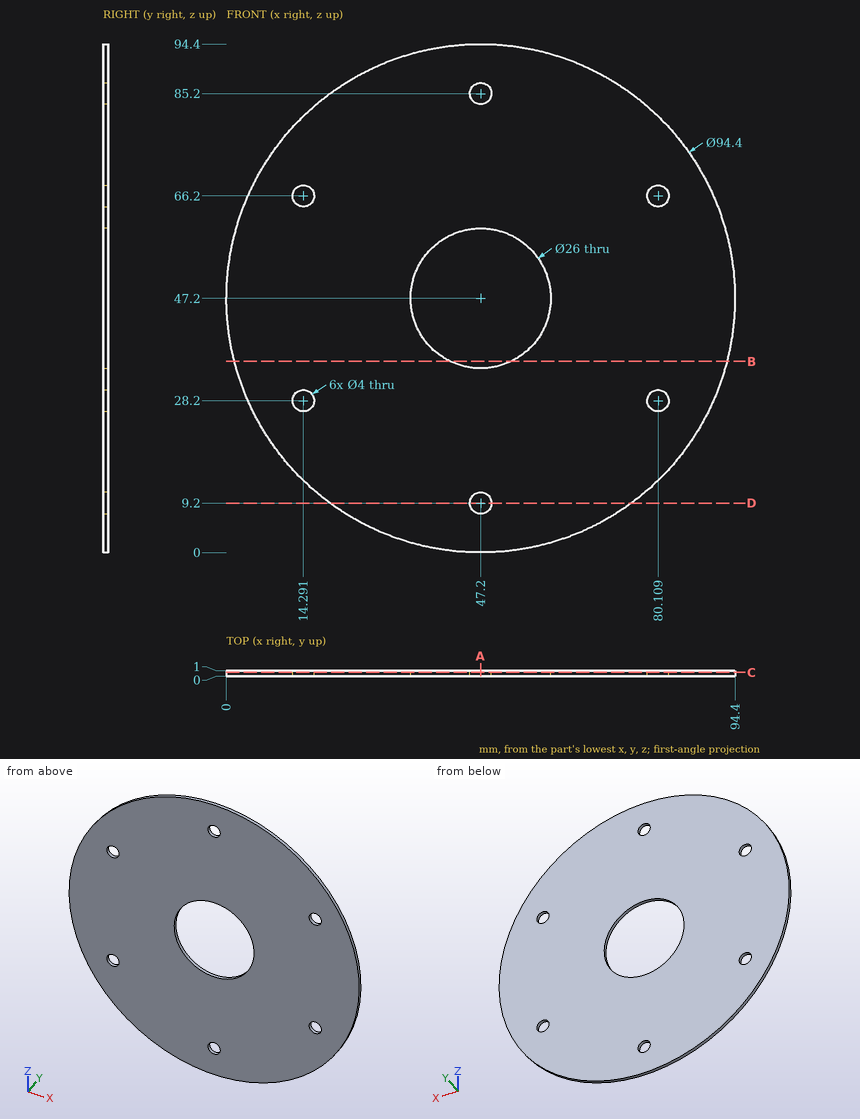
For this review, use the dimensioned drawing (mm, ordinates from the lowest corner) and the shaded views. Coordinates: 2 decimals unless noted, no trailing zeros. Loops run counter-clockwise (first coordinate to the right, second up) from the corner with the lowest first, then second, coordinate; pieces in that order, holes last. Notation, with made-up numbers: (60, 77.5) -> (88, 77.5) arc R22 cw to (88, 105.5) -> close; hole circle Ø3 at (81, 78.5). An arc over 180 degrees is marked (long way). Return JSON: item names as keys, results as strings. Group by question number.
(1) Consider section D-D, the plane z = 9.2. Give the boundary of the cut face in (x, y).
(2) Consider section A-A, the plane x = 47.2. Give the boundary of the cut face in (y, z).
(3) Consider section B-B, the plane z = 35.5. Give the boundary of the cut face in (x, y).
(4) Consider section C-C, the plane y = 0.65. Give the boundary of the cut face in (x, z).
(5) To check wall thickness, follow L1, parallel to X at y = 0.45, z = 28.2; L2, parallel to Z at x = 46.5, y = 0.6; L3, parallel to Z at x = 58, y = 0.25. State the ranges of each line that lie inside material, in increasing order.
Results below:
{
 "1": {"outline": "(19.2, 0) -> (45.2, 0) -> (45.2, 1) -> (19.2, 1) -> close; (49.2, 0) -> (75.2, 0) -> (75.2, 1) -> (49.2, 1) -> close"},
 "2": {"outline": "(0, 0) -> (1, 0) -> (1, 7.2) -> (0, 7.2) -> close; (0, 11.2) -> (1, 11.2) -> (1, 34.2) -> (0, 34.2) -> close; (0, 60.2) -> (1, 60.2) -> (1, 83.2) -> (0, 83.2) -> close; (0, 87.2) -> (1, 87.2) -> (1, 94.4) -> (0, 94.4) -> close"},
 "3": {"outline": "(1.47, 0) -> (41.53, 0) -> (41.53, 1) -> (1.47, 1) -> close; (52.87, 0) -> (92.93, 0) -> (92.93, 1) -> (52.87, 1) -> close"},
 "4": {"outline": "circle Ø94.4 at (47.2, 47.2); hole circle Ø4 at (14.29, 28.2); hole circle Ø4 at (14.29, 66.2); hole circle Ø26 at (47.2, 47.2); hole circle Ø4 at (47.2, 9.2); hole circle Ø4 at (47.2, 85.2); hole circle Ø4 at (80.11, 28.2); hole circle Ø4 at (80.11, 66.2)"},
 "5": {"L1": "x = 3.99 to 12.29, 16.29 to 78.11, 82.11 to 90.41", "L2": "z = 0.01 to 7.33, 11.07 to 34.22, 60.18 to 83.33, 87.07 to 94.39", "L3": "z = 1.25 to 39.96, 54.44 to 93.15"}
}
